```python
from build123d import *

# Parameters (mm, degrees)
F0_R     = 4
F1_DEPTH = 1
F2_R     = 3
F3_DEPTH = 10
F4_R     = 3
F5_W     = 2.2492834833
F5_H     = 10.7352328487
F5_W_2   = 1.4565391466
F6_DEPTH = 12.5
F7_R     = 1.1538217461
F8_DEPTH = 25


with BuildPart() as f1:
    # F0 (on Top) → F1 (new body)
    with BuildSketch(Plane.XY):
        Circle(F0_R)
    extrude(amount=F1_DEPTH)

    # F2 (on face) → F3 (join)
    with BuildSketch(Plane.XY.offset(1)):
        Circle(F2_R)
    extrude(amount=F3_DEPTH)

    # F4
    f4_edges = [f1.edges().sort_by_distance(p)[0] for p in [
        (-3, 0, 11),
    ]]
    fillet(f4_edges, radius=F4_R)

    # F5 (on Right) → F6 (cut, symmetric)
    with BuildSketch(Plane.YZ):
        with Locations((0, 8.051795885)):
            Rectangle(F5_W, F5_H)
        with Locations((-2.4088141508, 8.051795885)):
            Rectangle(F5_W_2, F5_H)
        with Locations((2.4088141508, 8.051795885)):
            Rectangle(F5_W_2, F5_H)
    extrude(amount=F6_DEPTH, both=True, mode=Mode.SUBTRACT)

    # F7 (on face) → F8 (cut)
    with BuildSketch(Plane(origin=(0, 1.6805445775, 0), x_dir=(-1, 0, 0), z_dir=(0, 1, 0))):
        with Locations((0, 8)):
            Circle(F7_R)
    extrude(amount=-F8_DEPTH, mode=Mode.SUBTRACT)


solid = f1.part
```
Geometry: final body of the model. Coordinates: model frame, mm. A direction names the side the tool comes from. Round coordinates to 2 decimals unless told otherwise and drop trailing zeros. Order: outer loops, then holes, each group sorted by start corner. A loop starts at its lowest first (then second) coordinate and runs counter-clockwise, first axis right, second up. Notation, with made-up numbers: M 37.5,24 L 43.5,24 A18 ccw 43.5,39 Z; hole C 86.25,42 d3. An arc over 180 degrees is marked long. One line per item, written item: value.
(1) Cut plane B-B (x = 0). Return the cut outline in (y, z).
Result sheet:
outline: M -4,0 L 4,0 L 4,1 L 3,1 L 3,2.68 L 1.68,2.68 L 1.68,6.85 L 1.12,6.85 L 1.12,2.68 L -1.12,2.68 L -1.12,6.85 L -1.68,6.85 L -1.68,2.68 L -3,2.68 L -3,1 L -4,1 Z; M -1.68,9.15 L -1.12,9.15 L -1.12,10.78 A3 ccw -1.68,10.49 Z; M 1.12,9.15 L 1.68,9.15 L 1.68,10.49 A3 ccw 1.12,10.78 Z
(2) Line query: probe 1 along Y at (x, z) = (2, 3.25); probe 2 along Z at (x, y) = (-1.5, -2.25); probe 3 along Y at (x, z) = (0, 1.25). Output: solid intervals per line, ascending. Write a range as [from, to].
Result sheet:
probe 1: [-1.68, -1.12], [1.12, 1.68]
probe 2: [0, 2.68]
probe 3: [-3, 3]
(3) Pull-direction query (Z, two-part tool) for faces 1 (the cylindrical face through (0.25, -1.399, 6.874)), 2 (the cylindrical face through (0.25, 1.406, 6.874)), 3 (the flat face through (0, -2, 2.684)), 4 (the cylindrical face through (-0.867, -3.905, 0.493)); classes: pulls with the +Z half, pulls with the -Z half, needs draft (parallel to the pull), parting line crosses it, or undercut.
Result sheet:
face 1: undercut
face 2: undercut
face 3: pulls with the +Z half
face 4: needs draft
(4) Reachability of faces 5 (the flat face through (0, 1.681, 6.5)), 6 (the flat face through (0, 0, 2.684)), 7 (the flat face through (0, -1.681, 6.5)), 8 (the flat face through (1, 3, 1)) from +Z, -Z, +X, -X, +Y, -Y: full face, straight path, thin tool, end or side. Return the list, or none.
Result sheet:
face 5: +Z, +X, -X, +Y
face 6: +Z, +X, -X
face 7: +Z, +X, -X, -Y
face 8: +Z
(5) Cut plane D-D (y = 1.25). Return the cut outline in (x, z).
Result sheet:
outline: M -3.8,0 L 3.8,0 L 3.8,1 L 2.73,1 L 2.73,8 A2.73 ccw -2.73,8 L -2.73,1 L -3.8,1 Z; hole C 0,8 d2.31
(6) Pin query (flat end, axial travel): P1, Ø1, axis at x = 2.5, z = 7.5, coming from the +Y side; P2, Ø3.5, axis at x = 0, z = 8, coming from the -Y side; P3, Ø1.8, axis at x = 0, z = 8, coming from the +Y side; P4, Ø1.8, axis at x = -0.5, y = -0.5, coming from the +Z side. Return the tip coordinate at first contact, or that it passes through.
Result sheet:
P1: y = 1.68
P2: y = -1.68
P3: through
P4: z = 10.78
(7) Cut plane C-C (y = 0). Return the cut outline in (x, z).
Result sheet:
outline: M -4,0 L 4,0 L 4,1 L 3,1 L 3,2.68 L -3,2.68 L -3,1 L -4,1 Z
(8) Cut plane A-A (z = 6.5). Return the cut outline in (x, y), and give its area (3 significant figures).
Result sheet:
outline: M -2.78,-1.12 A3 ccw -2.49,-1.68 L 2.49,-1.68 A3 ccw 2.78,-1.12 Z; M -2.78,1.12 L 2.78,1.12 A3 ccw 2.49,1.68 L -2.49,1.68 A3 ccw Z
area: 5.88 mm2
